Geometry check sheet. Reference: the model listing, model coordinates, mm. Face numbers are marked on the shaded views. Give positions to 0.01 mm unless a question says otherwise; leave off trailing zeros. Write each loop counter-clockwise with the first axis right and the second up, starting at its lowest first coordinate (ties: lowest second). Pieces come first, ordered by that corner, then holes. Notation, with made-up numbers: M 64.25,59.5 L 77.25,59.5 A23 cw 77.25,76.5 Z; hole C 15,75 d5. An arc over 180 degrees is marked long. Write each question's results on one line, items separated by ' | '.
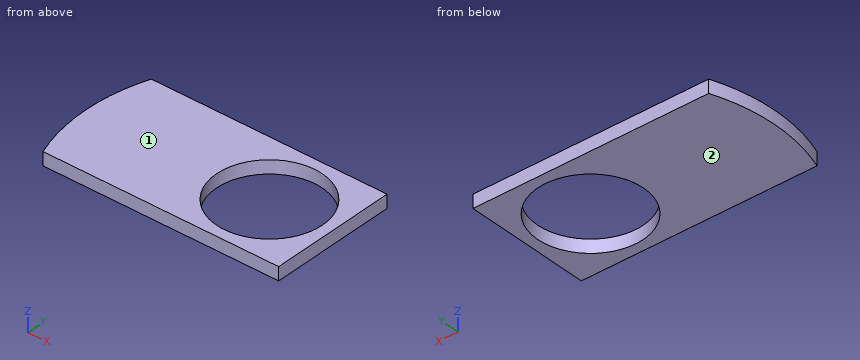
```python
from build123d import *

# Parameters (mm, degrees)
F0_R     = 2
F1_DEPTH = 0.5


with BuildPart() as f1:
    # F0 (on Top) → F1 (new body)
    with BuildSketch(Plane.XY):
        with BuildLine():
            Line((-5.986860613, 2.4), (-6.5224611919, 2.4))
            ThreePointArc((-6.5224611919, 2.4), (-6.95, 0), (-6.5224611919, -2.4))
            Line((-6.5224611919, -2.4), (-5.986860613, -2.4))
            ThreePointArc((-5.986860613, -2.4), (-6.45, 0), (-5.986860613, 2.4))
        make_face()
        with BuildLine():
            Line((2.4, -2.4), (2.4, 2.4))
            Line((2.4, 2.4), (-5.986860613, 2.4))
            ThreePointArc((-5.986860613, 2.4), (-6.45, 0), (-5.986860613, -2.4))
            Line((-5.986860613, -2.4), (2.4, -2.4))
        make_face()
        Circle(F0_R, mode=Mode.SUBTRACT)
    extrude(amount=F1_DEPTH)


solid = f1.part
```
Q1. Section check A-A (y = 0). Enter the section's corners in (x, z), then the cut area to 4 significant figures.
Answer key:
outline: M -6.95,0 L -2,0 L -2,0.5 L -6.95,0.5 Z; M 2,0 L 2.4,0 L 2.4,0.5 L 2,0.5 Z | area: 2.675 mm2
Q2. Section check B-B (x = 0). Enter the section's corners in (y, z), then the cut area to 3 significant figures.
Answer key:
outline: M -2.4,0 L -2,0 L -2,0.5 L -2.4,0.5 Z; M 2,0 L 2.4,0 L 2.4,0.5 L 2,0.5 Z | area: 0.400 mm2
Q3. Material ranges on probe 1 along Y at (x, z) = (0, 0.4); probe 2 along X at (y, z) = (-0.9, 0.3); probe 3 along X at (y, z) = (0.75, 0.4), recorded low to high. Write a range as [from, to].
Answer key:
probe 1: y = [-2.4, -2], [2, 2.4] | probe 2: x = [-6.89, -1.79], [1.79, 2.4] | probe 3: x = [-6.91, -1.85], [1.85, 2.4]
Q4. Section check C-C (z = 0.1). Enter the section's corners in (x, y).
Answer key:
outline: M -6.52,-2.4 L 2.4,-2.4 L 2.4,2.4 L -6.52,2.4 A6.95 ccw Z; hole C 0,0 d4
Q5. Release check for a two-part mould opening along Z. For the marked faces 1 and 2 record: released by +Z, released by -Z, zero draft, split by the parting line, or undercut.
Answer key:
face 1: released by +Z | face 2: released by -Z
Q6. Section check D-D (y = -2.1). Enter the section's corners in (x, z), then the cut area to 3 significant figures.
Answer key:
outline: M -6.63,0 L 2.4,0 L 2.4,0.5 L -6.63,0.5 Z | area: 4.51 mm2
